CAD build for the part. Positions are in the model's coordinates, mm. Face numbers are marked on the shaded views. A direction names the side the tool comes from. Give positions to 0.01 mm unless a question says otherwise; leave off trailing zeros. Order: outer loops, then holes, each group sorted by start corner. A loop starts at its lowest first (then second) coordinate and runs counter-clockwise, first axis right, second up. Notation, with made-up numbers: (61, -36) -> (87, -36) arc R5 cw to (87, -29) -> close; hole circle Ø9 at (-35.5, 72). An arc over 180 degrees is marked (long way). Answer as CSV lines item,"result".
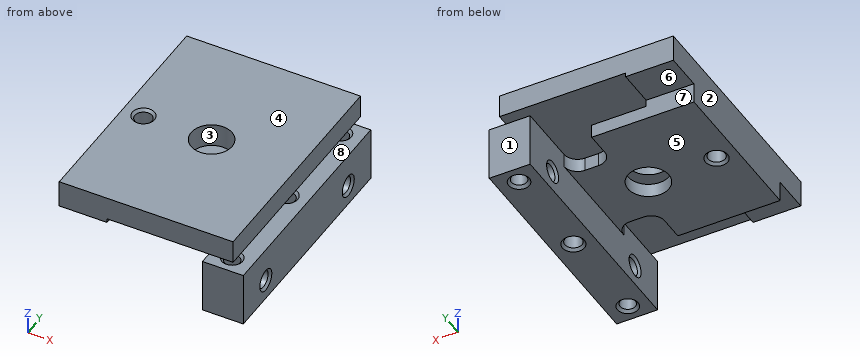
```python
from build123d import *

# Parameters (mm, degrees)
SKETCH_1_W                   = 27
SKETCH_1_H                   = 34
EXTRUDE_1_DEPTH              = 13
SKETCH_2_W                   = 20
SKETCH_2_H                   = 1.6
CUT_EXTRUDE_1_DEPTH          = 46.321076774
CUT_EXTRUDE_2_DEPTH          = 9
CUT_EXTRUDE_3_REACH          = 47.321
SKETCH_4_W                   = 1.5
SKETCH_4_H                   = 34
SKETCH_12_W                  = 21
SKETCH_12_H                  = 34
CUT_EXTRUDE_7_DEPTH          = 6
SKETCH_8_R                   = 3
CUT_EXTRUDE_4_DEPTH          = 46.321076774
HOLE_WIZARD_M31_AT_2_COUNT   = 2
HOLE_WIZARD_M31_AT_2_PITCH   = 22
HOLE_WIZARD_4_401_AT_2_COUNT = 2
HOLE_WIZARD_4_401_AT_2_PITCH = 29


# Read off the part's stored shape, not the designer's step: Отверстие обработанное метчиком M3x0.52
with BuildPart() as part:
    # Эскиз1 → Вытянуть1 (new body)
    with BuildSketch(Plane.XY):
        with Locations((13.5, 17)):
            Rectangle(SKETCH_1_W, SKETCH_1_H)
    extrude(amount=EXTRUDE_1_DEPTH)

    # Эскиз2 → Вырез-Вытянуть1 (cut, through all)
    with BuildSketch(Plane(origin=(0, 34, 0), x_dir=(1, 0, 0), z_dir=(0, 1, 0))):
        with Locations((17, -8.8)):
            Rectangle(SKETCH_2_W, SKETCH_2_H)
    extrude(amount=-CUT_EXTRUDE_1_DEPTH, mode=Mode.SUBTRACT)

    # Эскиз3 → Вырез-Вытянуть2 (cut)
    with BuildSketch(Plane(origin=(0, 0, 0), x_dir=(-1, 0, 0), z_dir=(0, 0, -1))):
        with BuildLine():
            Line((0, 34), (-21, 34))
            Line((-21, 34), (-21, 25))
            ThreePointArc((-21, 25), (-20.414213562, 23.585786438), (-19, 23))
            Line((-19, 23), (-17, 23))
            ThreePointArc((-17, 23), (-15.585786438, 23.585786438), (-15, 25))
            Line((-15, 25), (-15, 28.5))
            Line((-15, 28.5), (0, 28.5))
            Line((0, 28.5), (0, 34))
        make_face()
        with BuildLine():
            Line((0, 0), (0, 5.5))
            Line((0, 5.5), (-15, 5.5))
            Line((-15, 5.5), (-15, 9))
            ThreePointArc((-15, 9), (-15.585786438, 10.414213562), (-17, 11))
            Line((-17, 11), (-19, 11))
            ThreePointArc((-19, 11), (-20.414213562, 10.414213562), (-21, 9))
            Line((-21, 9), (-21, 0))
            Line((-21, 0), (0, 0))
        make_face()
    extrude(amount=-CUT_EXTRUDE_2_DEPTH, mode=Mode.SUBTRACT)

    # Эскиз4 → Вырез-Вытянуть3 (cut, up to next)
    with BuildSketch(Plane.XY.offset(13), mode=Mode.PRIVATE) as cut_extrude_3_sk1:
        with Locations((26.25, 17)):
            Rectangle(SKETCH_4_W, SKETCH_4_H)
    cut_extrude_3_tool1 = extrude(cut_extrude_3_sk1.sketch, amount=-CUT_EXTRUDE_3_REACH, mode=Mode.PRIVATE) & part.part
    add(cut_extrude_3_tool1.solids().sort_by_distance((26.25, 17, 13))[0], mode=Mode.SUBTRACT)

    # Эскиз12 → Вырез-Вытянуть7 (cut)
    with BuildSketch(Plane(origin=(0, 0, 0), x_dir=(-1, 0, 0), z_dir=(0, 0, -1))):
        with Locations((-10.5, 17)):
            Rectangle(SKETCH_12_W, SKETCH_12_H)
    extrude(amount=-CUT_EXTRUDE_7_DEPTH, mode=Mode.SUBTRACT)

    # Эскиз8 → Вырез-Вытянуть4 (cut, through all)
    with BuildSketch(Plane(origin=(0, 0, 0), x_dir=(-1, 0, 0), z_dir=(0, 0, -1))):
        with Locations((-13, 17)):
            Circle(SKETCH_8_R)
    extrude(amount=-CUT_EXTRUDE_4_DEPTH, mode=Mode.SUBTRACT)

    # Эскиз19 → Отверстие обработанное метчиком M31 (revolve, cut)
    with BuildSketch(Plane(origin=(27, 28, 3), x_dir=(0, 0, -1), z_dir=(0, 1, 0))):
        Polygon((0, 0), (0, 6), (1.6, 6), (1.25, 5.65), (1.25, 0.35), (1.6, 0), align=None)
    hole_wizard_m31 = revolve(axis=Axis((33.35, 28, 3), (-1, 0, 0)), mode=Mode.SUBTRACT)

    # Отверстие обработанное метчиком M31 at 2: Отверстие обработанное метчиком M31 ×2
    with Locations(*[(0, -i * HOLE_WIZARD_M31_AT_2_PITCH, 0) for i in range(1, HOLE_WIZARD_M31_AT_2_COUNT)]):
        add(hole_wizard_m31, mode=Mode.SUBTRACT)

    # Отверстие обработанное метчиком M3x0.52 outline → Отверстие обработанное метчиком M3x0.52 (revolve, cut)
    with BuildSketch(Plane(origin=(24, 17, 0), x_dir=(1, 0, 0), z_dir=(0, -1, 0))):
        Polygon((1.625, 8), (0, 8), (0, 0), (1.625, 0), (1.25, 0.375), (1.25, 7.625), align=None)
    revolve(axis=Axis((24, 17, 0), (0, 0, 1)), mode=Mode.SUBTRACT)

    # M3x0.52 2 outline → M3x0.52 2 (revolve, cut)
    with BuildSketch(Plane(origin=(3, 17, 0), x_dir=(1, 0, 0), z_dir=(0, -1, 0))):
        Polygon((1.625, 13), (0, 13), (0, 6), (1.625, 6), (1.25, 6.375), (1.25, 12.625), align=None)
    revolve(axis=Axis((3, 17, 0), (0, 0, 1)), mode=Mode.SUBTRACT)

    # Эскиз24 → Отверстие обработанное метчиком #4-401 (revolve, cut)
    with BuildSketch(Plane(origin=(24, 2.5, 0), x_dir=(0, 1, 0), z_dir=(1, 0, 0))):
        Polygon((0, 0), (0, 8), (1.524, 8), (1.1303, 7.6063), (1.1303, 0.3937), (1.524, 0), align=None)
    hole_wizard_4_401 = revolve(axis=Axis((24, 2.5, -6.35), (0, 0, 1)), mode=Mode.SUBTRACT)

    # Отверстие обработанное метчиком #4-401 at 2: Отверстие обработанное метчиком #4-401 ×2
    with Locations(*[(0, i * HOLE_WIZARD_4_401_AT_2_PITCH, 0) for i in range(1, HOLE_WIZARD_4_401_AT_2_COUNT)]):
        add(hole_wizard_4_401, mode=Mode.SUBTRACT)


solid = part.part
```
1) Band-saw the part on D-D, the plane y = 26. Write the cut outline in (x, z), then the cut area to 3 significant figures.
Data:
outline,"(0, 6) -> (15, 6) -> (15, 8) -> (7, 8) -> (7, 9.6) -> (25.5, 9.6) -> (25.5, 13) -> (0, 13) -> close; (21, 0) -> (27, 0) -> (27, 8) -> (21, 8) -> close"
area,"176 mm2"
2) Band-saw the part on B-B, the plane x = 24. Give the number of separate pieces and of enclosed holes in the cut face, then the cut area to 3 significant figures.
Data:
separate pieces,"5"
enclosed holes,"2"
area,"321 mm2"
3) Wall check: line 1 along Z through (x, y) = (25, 6); line 2 along Y through (x, z) = (3, 11); line 3 along Z through (x, y) = (21.75, 4). Give the ranges that are in metal, low to high. Write a range as [from, to].
Data:
line 1,"z = [0, 1.75], [4.25, 8], [9.6, 13]"
line 2,"y = [0, 15.75], [18.25, 34]"
line 3,"z = [0, 8], [9.6, 13]"
4) Pull direction X, two halves, no side cores. Call the marked faces 1, 2 and 3: pulls with the +X half, pulls with the -X half, needs draft (parallel to the pull), parting line crosses it, or undercut.
Data:
face 1,"needs draft"
face 2,"pulls with the -X half"
face 3,"undercut"
5) Band-saw the part on C-C, the plane y = 31.5. Write the cut outline in (x, z).
Data:
outline,"(0, 9) -> (7, 9) -> (7, 9.6) -> (25.5, 9.6) -> (25.5, 13) -> (0, 13) -> close; (21, 0) -> (22.48, 0) -> (22.87, 0.39) -> (22.87, 7.61) -> (22.48, 8) -> (21, 8) -> close; (25.13, 0.39) -> (25.52, 0) -> (27, 0) -> (27, 8) -> (25.52, 8) -> (25.13, 7.61) -> close"
6) Which spindle directions (+Z, -Z, +X, -X, +Y, -Y) get a long thin tool onto all of the face, cutting with end or side? Do the marked faces 4, 5, 6, 7 and 8. Say none if no direction does.
Data:
face 4,"+Z, +X, -X, +Y, -Y"
face 5,"-Z, -X, +Y, -Y"
face 6,"-Z, +X, -X, +Y"
face 7,"-Z, -X, +Y"
face 8,"+X, +Y, -Y"
7) Band-saw the part on A-A, the plane z = 3. Write the cut outline in (x, y).
Data:
outline,"(21, 0) -> (27, 0) -> (27, 4.4) -> (26.65, 4.75) -> (21.35, 4.75) -> (21, 4.4) -> close; (21, 7.6) -> (21.35, 7.25) -> (26.65, 7.25) -> (27, 7.6) -> (27, 26.4) -> (26.65, 26.75) -> (21.35, 26.75) -> (21, 26.4) -> close; (21, 29.6) -> (21.35, 29.25) -> (26.65, 29.25) -> (27, 29.6) -> (27, 34) -> (21, 34) -> close; hole circle Ø2.5 at (24, 17); hole circle Ø2.26 at (24, 2.5); hole circle Ø2.26 at (24, 31.5)"
8) Pin check, flat tips, straight feed: P1, Ø1.5, axis at y = 6, z = 3, coming from the +X side; P2, Ø9.5, axis at x = 13, y = 17, coming from the -Z side; P3, Ø3.5, axis at x = 4, z = 7.5, coming from the +Y side; P4, Ø1.6, axis at x = 2, y = 31.5, coming from the -Z side. Stop position of each tip, or through.
Data:
P1,"passes through"
P2,"stops at z = 6"
P3,"stops at y = 34"
P4,"stops at z = 9"
